The listing builds one solid part. Answer for the finished solid, in the listing's coordinates (mm). A direction names the side the tool comes from. Give positions to 0.01 mm unless a question says otherwise; leave off trailing zeros. Loops run counter-clockwise (first coordinate to the right, second up) from the corner with the lowest first, then second, coordinate; pieces in that order, holes last. Notation, with made-up numbers: M -26.5,7 L 14.5,7 A25 ccw 14.5,24 Z; hole C -36.5,-31 d1. An arc over 180 degrees is marked long. One line per item, written item: value. Start each with the question number.
Q1. A cutting plane is placed at B-B, the plane z = 0. Determine the outline of the cut face in (x, y), and give its area (3 significant figures).
Q2. Consider L1, parallel to Z at x = 0, y = 1.6; L2, parallel to X at y = 8.25, z = -21.5; L3, parallel to Z at x = -23, y = 7.25. Determine where each line is inside the solid, lowest interval first.
Q3. A cutting plane is placed at C-C, the plane y = 1.25. Determine the outline of the cut face in (x, z).
Q4. The mould has two halves that part along Z. Classify faces 1 (the flat face through (-22, 0, -31)), 2 (the cylindrical face through (1.5, 1.48, -0.07)), 3 (the flat face through (-23, 1, -65.5)): +Z half, -Z half, draft (parallel to the pull), parting line (faces both ways), or undercut.
Q5. A cutting plane is placed at A-A, the plane x = -45. Determine the outline of the cut face in (y, z), and give its area (3 significant figures).
Q6. For faces 4 (the flat face through (-47.5, 1, -31)), 5 (the flat face through (-7.5, 6, -31)), 6 (the flat face through (-22, 6, -55.5)), determine the directions among +Z, -Z, +X, -X, +Y, -Y from which every point of the face is accessible in a straight line to the end or side of a thin tool.
Q7. Flat-ended cylindrical pins translate along their axes: pin 1 (4 mm diameter, centred on x = -40.5, z = -8.5, fed in from -Y); pin 2 (1.8 mm diameter, centred on x = -45, z = -45, fed in from -Y); pin 3 (1 mm diameter, centred on x = -7.5, y = 7.5, fed in from +Z); pin 4 (3.5 mm diameter, centred on x = -32, y = 1.5, fed in from -Z). Find the tip coordinate at first contact, or state that the pin passes through.
Q8. A cutting plane is placed at D-D, the plane z = -30. Determine the outline of the cut face in (x, y).
Autodesk Inventor part; units mm, degrees
ref_plane "YZ Plane" through (0, 0, 0) normal (1, 0, 0) x (0, 1, 0)
ref_plane "XZ Plane" through (0, 0, 0) normal (0, 1, 0) x (-1, 0, 0)
ref_plane "XY Plane" through (0, 0, 0) normal (0, 0, 1) x (1, 0, 0)
sketch "Sketch1" plane through (0, 0, 0) normal (0, 1, 0) x (-1, 0, 0)
  line L0 (0, 0) -> (45, 0) construction
  line L1 (45, 0) -> (45, -45) construction
  line L2 (45, -45) -> (0, -45) construction
  line L3 (0, -45) -> (0, 0) construction
  circle A0 centre (45, 0) radius 1.5
  circle A1 centre (45, -45) radius 1.5
  circle A2 centre (0, -45) radius 1.5
  circle A3 centre (0, 0) radius 1.5
  line L4 (-2.5, 2.5) -> (47.5, 2.5)
  line L5 (47.5, 2.5) -> (47.5, -65.5)
  line L6 (47.5, -65.5) -> (-2.5, -65.5)
  line L7 (-2.5, -65.5) -> (-2.5, 2.5)
  dimension "d0" = 45
  dimension "d1" = 45
  dimension "d2" = 3
  dimension "d3" = 3
  dimension "d4" = 3
  dimension "d5" = 3
  dimension "d6" = 50
  dimension "d7" = 68
  dimension "d8" = 2.5
  dimension "d9" = 2.5
extrude "Extrusion1" add sketch "Sketch1" along normal blind 3
sketch "Sketch2" plane through (0, 3, 0) normal (0, 1, 0) x (1, 0, 0)
  line L0 (2.5, -2.5) -> (2.5, 65.5)
  line L1 (2.5, 40.5) -> (-7.5, 40.5)
  line L2 (-7.5, 40.5) -> (-7.5, 20.5)
  line L3 (-7.5, 20.5) -> (2.5, 20.5)
  line L4 (2.5, 20.5) -> (2.5, 40.5)
  line L5 (2.5, 65.5) -> (-47.5, 65.5)
  line L6 (-47.5, 65.5) -> (-47.5, -2.5)
  line L7 (-47.5, 40.5) -> (-37.5, 40.5)
  line L8 (-37.5, 40.5) -> (-37.5, 20.5)
  line L9 (-37.5, 20.5) -> (-47.5, 20.5)
  line L10 (-47.5, 20.5) -> (-47.5, 40.5)
  line L11 (-26.5, 65.5) -> (-18.5, 65.5)
  line L12 (-18.5, 65.5) -> (-18.5, 55.5)
  line L13 (-18.5, 55.5) -> (-26.5, 55.5)
  line L14 (-26.5, 55.5) -> (-26.5, 65.5)
  point P0 (0, 0)
  point P1 (2.5, 20.5)
  dimension "d12" = 10
  dimension "d13" = 20
  dimension "d14" = 25
  dimension "d15" = 10
  dimension "d16" = 20
  dimension "d19" = 8
  dimension "d20" = 10
  dimension "d21" = 50
  dimension "d22" = 68
  dimension "d23" = 21
extrude "Extrusion2" add sketch "Sketch2" along normal blind 7
sketch "Sketch3" plane through (2.5, 0, 2.5) normal (1, 0, 0) x (0, 0, -1)
  line L0 (43, 10) -> (23, 10)
  line L1 (43, 3) -> (23, 3)
  line L2 (23, 10) -> (43, 10)
  line L3 (43, 10) -> (43, 3)
  line L4 (43, 3) -> (23, 3)
  line L5 (23, 3) -> (23, 10)
  point P0 (2.5, 0)
extrude "Extrusion3" add sketch "Sketch3" along normal blind 10
sketch "Sketch4" plane through (-47.5, 0, -65.5) normal (-1, 0, 0) x (0, 0, 1)
  line L0 (25, 3) -> (25, 10)
  line L1 (45, 3) -> (45, 10)
  line L2 (25, 10) -> (45, 10)
  line L3 (45, 10) -> (45, 3)
  line L4 (45, 3) -> (25, 3)
  line L5 (25, 3) -> (25, 10)
  point P0 (65.5, 0)
extrude "Extrusion4" add sketch "Sketch4" along normal blind 10
sketch "Sketch5" plane through (2.5, 0, -65.5) normal (0, 0, -1) x (-1, 0, 0)
  line L0 (21, 10) -> (29, 10)
  line L1 (29, 3) -> (50, 3)
  line L2 (21, 10) -> (29, 10)
  line L3 (29, 10) -> (29, 3)
  line L4 (29, 3) -> (21, 3)
  line L5 (21, 3) -> (21, 10)
  point P0 (2.5, 0)
extrude "Extrusion5" add sketch "Sketch5" along normal blind 10
equation "\"d8\" = -0.5 * d0 + 0.5 * d6"
equation "\"d9\" = d8"
equation "\"d23\" = -0.5 * d19 + 0.5 * d21"
properties part number "Holybro PM07 PowerDistributionBoard"
Answer block:
1. outline: M -47.5,0 L -46.5,0 L -46.5,3 L -47.5,3 Z; M -43.5,0 L -1.5,0 L -1.5,3 L -43.5,3 Z; M 1.5,0 L 2.5,0 L 2.5,3 L 1.5,3 Z
1. area: 132 mm^2
2. L1: -65.5 to -46.5, -43.5 to -1.5, 1.5 to 2.5
2. L2: -57.5 to -37.5, -7.5 to 12.5
2. L3: -75.5 to -55.5
3. outline: M -47.5,-65.5 L 2.5,-65.5 L 2.5,2.5 L -47.5,2.5 Z; hole C -45,-45 d3; hole C -45,0 d3; hole C 0,-45 d3; hole C 0,0 d3
4. face 1: draft
4. face 2: undercut
4. face 3: -Z half
5. outline: M 0,-65.5 L 3,-65.5 L 3,-46.5 L 0,-46.5 Z; M 0,-43.5 L 3,-43.5 L 3,-40.5 L 10,-40.5 L 10,-20.5 L 3,-20.5 L 3,-1.5 L 0,-1.5 Z; M 0,1.5 L 3,1.5 L 3,2.5 L 0,2.5 Z
5. area: 326 mm^2
6. face 4: +Z, -Z, -X, -Y
6. face 5: +Z, -Z, +Y
6. face 6: +Z, +X, -X, +Y
7. pin 1: y = 0
7. pin 2: through
7. pin 3: z = -20.5
7. pin 4: z = -65.5
8. outline: M -57.5,3 L -47.5,3 L -47.5,0 L 2.5,0 L 2.5,3 L 12.5,3 L 12.5,10 L -7.5,10 L -7.5,3 L -37.5,3 L -37.5,10 L -57.5,10 Z
